Part model, mm, in its own coordinate system. A direction names the side the tool comes from. Round coordinates to 2 decimals unless told otherwise and drop trailing zeros. Write each loop counter-clockwise with the first axis right and the second up, starting at its lowest first coordinate (ties: lowest second). Pieces come first, ordered by that corner, then holes.
from build123d import *

# Parameters (mm, degrees)
F0_W     = 127
F0_H     = 50.8
F1_DEPTH = 25.4
F2_SIZE  = 5.08
F3_R     = 5.08
F4_W     = 111.76
F4_H     = 35.56
F5_DEPTH = 8.89
F6_R     = 5.08


with BuildPart() as f1:
    # F0 (on Top) → F1 (new body)
    with BuildSketch(Plane.XY):
        Rectangle(F0_W, F0_H)
    extrude(amount=F1_DEPTH)

    # F2
    f2_edges = [f1.edges().sort_by_distance(p)[0] for p in [
        (-63.5, -25.4, 12.7),
    ]]
    chamfer(f2_edges, length=F2_SIZE)

    # F3
    f3_edges = [f1.edges().sort_by_distance(p)[0] for p in [
        (63.5, -25.4, 12.7),
    ]]
    fillet(f3_edges, radius=F3_R)

    # F4 (on face) → F5 (cut)
    with BuildSketch(Plane.XY.offset(25.4)):
        Rectangle(F4_W, F4_H)
    extrude(amount=-F5_DEPTH, mode=Mode.SUBTRACT)

    # F6
    f6_edges = [f1.edges().sort_by_distance(p)[0] for p in [
        (0, 17.78, 16.51),
        (-55.88, 0, 16.51),
        (0, -17.78, 16.51),
        (55.88, 0, 16.51),
        (-55.88, 17.78, 20.955),
        (-55.88, -17.78, 20.955),
        (55.88, -17.78, 20.955),
        (55.88, 17.78, 20.955),
    ]]
    fillet(f6_edges, radius=F6_R)


solid = f1.part
Q1. Saw through at A-A, the plane y = -1. Write the cut outline in (x, z), and give its area (3 significant figures).
Q2. Saw through at B-B, the plane x = 1.5. Write the cut outline in (y, z).
Q3. Wall check: line 1 (X direction, y = -10.5, z = 22.25); line 2 (Y direction, x = -47.5, z = 22.5); line 3 (Z direction, x = 12, y = 6). Give the ranges that are in metal, low to high.
Q4. Tool access for faces 4 (the flat face through (-1, -25.4, 13)), 5 (the cylindrical face through (-54.431, 0.178, 18.038)): list every direction of +Z, -Z, +X, -X, +Y, -Y with a clear straight run to the whole face (end or side of a thin tool).
Q5. Two-plate mould, pull along Y, no slides. Class faces 1 (the flat face through (63.5, 2, 13)), 2 (the cylindrical face through (-54.352, 16.331, 23.468)), 3 (the cylindrical face through (61.972, -23.951, 12.878)): released by +Y, released by -Y, zero draft, split by the parting line, or undercut.
Q6. Drop flat-ended pins along their axis: P1, Ø20.5, axis at x = -24, y = -3, coming from the +Z side; P2, Ø4, axis at x = -46, y = 12, coming from the +Z side. Give the stop position or say it passes through.
Computed:
1. outline: (-63.5, 0) - (63.5, 0) - (63.5, 25.4) - (55.88, 25.4) - (55.88, 21.59) arc R5.08 cw to (50.8, 16.51) - (-50.8, 16.51) arc R5.08 cw to (-55.88, 21.59) - (-55.88, 25.4) - (-63.5, 25.4) - close
1. area: 2,240 mm2
2. outline: (-25.4, 0) - (25.4, 0) - (25.4, 25.4) - (17.78, 25.4) - (17.78, 21.59) arc R5.08 cw to (12.7, 16.51) - (-12.7, 16.51) arc R5.08 cw to (-17.78, 21.59) - (-17.78, 25.4) - (-25.4, 25.4) - close
3. line 1: x = -63.5 to -55.88, 55.88 to 63.5
3. line 2: y = -25.4 to -17.78, 17.78 to 25.4
3. line 3: z = 0 to 16.51
4. face 4: +Z, -Z, +X, -X, -Y
4. face 5: +Z
5. face 1: zero draft
5. face 2: undercut
5. face 3: released by -Y
6. P1: stops at z = 16.54
6. P2: stops at z = 16.68
